from build123d import *

# Parameters (mm, degrees)
SKETCH_1_W          = 120
SKETCH_1_H          = 75
SKETCH_1_W_2        = 114
SKETCH_1_H_2        = 69
EXTRUDE_1_DEPTH     = 45
SKETCH_2_W          = 114
SKETCH_2_H          = 69
SKETCH_2_R          = 30
EXTRUDE_2_DEPTH     = 4
CUT_EXTRUDE_1_DEPTH = 84.852549156
SKETCH_3_W          = 8
SKETCH_3_H          = 8
EXTRUDE_3_DEPTH     = 3
SKETCH_3_3_R        = 0.9
CUT_EXTRUDE_2_DEPTH = 3
SKETCH_4_R          = 5.5
CUT_EXTRUDE_3_DEPTH = 2


with BuildPart() as part:
    # Sketch 1 → Extrude 1 (new body)
    with BuildSketch(Plane.XY):
        Rectangle(SKETCH_1_W, SKETCH_1_H)
        Rectangle(SKETCH_1_W_2, SKETCH_1_H_2, mode=Mode.SUBTRACT)
    extrude(amount=EXTRUDE_1_DEPTH)

    # Sketch 2 → Extrude 2 (add)
    with BuildSketch(Plane.XY.offset(45)):
        Rectangle(SKETCH_2_W, SKETCH_2_H)
        with Locations((-20, 0)):
            Circle(SKETCH_2_R, mode=Mode.SUBTRACT)
    extrude(amount=-EXTRUDE_2_DEPTH)

    # Sketch 2_4 → Cut-Extrude 1 (cut, through all)
    with BuildSketch(Plane.XY.offset(45)):
        with BuildLine():
            ThreePointArc((12.841478126, 8.799847414), (9.44486376, 16.999999947), (4.04163056, 24.04163056))
            ThreePointArc((4.04163056, 24.04163056), (2.415284962, 24.041630558), (2.415284968, 22.41528496))
            ThreePointArc((2.415284968, 22.41528496), (7.453005293, 15.850000012), (10.619848685, 8.204563761))
            ThreePointArc((10.619848685, 8.204563761), (12.02830522, 7.391390911), (12.841478126, 8.799847414))
        make_face()
        with BuildLine():
            ThreePointArc((-28.799847612, -32.841478073), (-20, -34), (-11.200152388, -32.841478073))
            ThreePointArc((-11.200152388, -32.841478073), (-10.386979697, -31.433021385), (-11.795436406, -30.61984873))
            ThreePointArc((-11.795436406, -30.61984873), (-20.000000038, -31.7), (-28.204563667, -30.61984871))
            ThreePointArc((-28.204563667, -30.61984871), (-29.613020313, -31.433021421), (-28.799847612, -32.841478073))
        make_face()
        with BuildLine():
            ThreePointArc((-44.04163056, 24.04163056), (-49.444863704, 17.000000043), (-52.841478068, 8.79984763))
            ThreePointArc((-52.841478068, 8.79984763), (-52.028305318, 7.391390937), (-50.61984868, 8.204563781))
            ThreePointArc((-50.61984868, 8.204563781), (-47.453005293, 15.850000012), (-42.415284981, 22.415284946))
            ThreePointArc((-42.415284981, 22.415284946), (-42.415284955, 24.041630551), (-44.04163056, 24.04163056))
        make_face()
    extrude(amount=-CUT_EXTRUDE_1_DEPTH, mode=Mode.SUBTRACT)

    # Sketch 3 → Extrude 3 (add)
    with BuildSketch(Plane(origin=(0, 0, 0), x_dir=(-1, 0, 0), z_dir=(0, 0, -1))):
        with Locations((-56, 33.5)):
            Rectangle(SKETCH_3_W, SKETCH_3_H)
        with Locations((56, 33.5)):
            Rectangle(SKETCH_3_W, SKETCH_3_H)
        with Locations((-56, -33.5)):
            Rectangle(SKETCH_3_W, SKETCH_3_H)
        with Locations((56, -33.5)):
            Rectangle(SKETCH_3_W, SKETCH_3_H)
    extrude(amount=-EXTRUDE_3_DEPTH)

    # Sketch 3_3 → Cut-Extrude 2 (cut)
    with BuildSketch(Plane(origin=(0, 0, 0), x_dir=(-1, 0, 0), z_dir=(0, 0, -1))):
        with Locations((-56, 33.5)):
            Circle(SKETCH_3_3_R)
        with Locations((-56, -33.5)):
            Circle(SKETCH_3_3_R)
        with Locations((56, -33.5)):
            Circle(SKETCH_3_3_R)
        with Locations((56, 33.5)):
            Circle(SKETCH_3_3_R)
    extrude(amount=-CUT_EXTRUDE_2_DEPTH, mode=Mode.SUBTRACT)

    # Sketch 4 → Cut-Extrude 3 (cut)
    with BuildSketch(Plane.XY.offset(45)):
        with Locations((40, 18)):
            Circle(SKETCH_4_R)
        with Locations((40, 0)):
            Circle(SKETCH_4_R)
        with Locations((40, -18)):
            Circle(SKETCH_4_R)
    extrude(amount=-CUT_EXTRUDE_3_DEPTH, mode=Mode.SUBTRACT)


solid = part.part
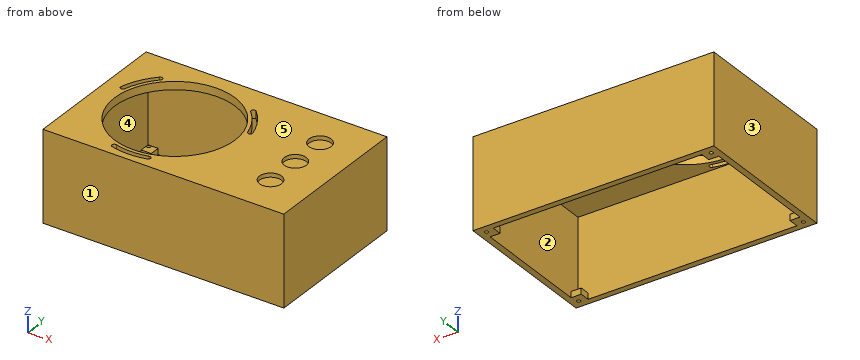
Verification items for the finished model (mm, model axes). Face numbers are marked on the shaded views. A direction names the side the tool comes from. Coordinates: 2 decimals unless noted, no trailing zeros. Order: outer loops, then holes, each group sorted by start corner. A loop starts at its lowest first (then second) coordinate and runs counter-clockwise, first axis right, second up.
Item 1: Access from +Z, -Z, +X, -X, +Y, -Y to the whole of each face (thin tool, end or side, straight path). Record for the marked faces 1 and 2.
Filled in:
face 1: +Z, -Z, +X, -X, -Y
face 2: none
Item 2: Release check for a two-part mould opening along X. For the marked faces 3, 4 and 5 record: +X half, -X half, draft (parallel to the pull), parting line (faces both ways), or undercut.
Filled in:
face 3: -X half
face 4: undercut
face 5: draft
Item 3: Section check D-D, the plane y = 18. Enter the section's corners in (x, z).
Filled in:
outline: (-60, 0) - (-57, 0) - (-57, 41) - (-48.84, 41) - (-48.84, 45) - (-60, 45) - close; (-46.09, 41) - (-44, 41) - (-44, 45) - (-46.09, 45) - close; (4, 41) - (6.09, 41) - (6.09, 45) - (4, 45) - close; (8.84, 41) - (57, 41) - (57, 0) - (60, 0) - (60, 45) - (45.5, 45) - (45.5, 43) - (34.5, 43) - (34.5, 45) - (8.84, 45) - close
Item 4: Section check B-B, the plane z = 33. Enter the section's corners in (x, y).
Filled in:
outline: (-60, -37.5) - (60, -37.5) - (60, 37.5) - (-60, 37.5) - close; hole (-57, -34.5) - (57, -34.5) - (57, 34.5) - (-57, 34.5) - close
Item 5: Material ranges on L1, parallel to Y at x = 40, z = 44; L2, parallel to X at y = 33.5, z = 1.2; L3, parallel to Y at x = -56, z = 2.4, recorded low to high.
Filled in:
L1: y = -37.5 to -23.5, -12.5 to -5.5, 5.5 to 12.5, 23.5 to 37.5
L2: x = -60 to -56.9, -55.1 to -52, 52 to 55.1, 56.9 to 60
L3: y = -37.5 to -34.4, -32.6 to -29.5, 29.5 to 32.6, 34.4 to 37.5
Item 6: Section check C-C, the plane x = -47. Enter the section's corners in (y, z).
Filled in:
outline: (-37.5, 0) - (-34.5, 0) - (-34.5, 41) - (-13.08, 41) - (-13.08, 45) - (-37.5, 45) - close; (13.08, 41) - (16.61, 41) - (16.61, 45) - (13.08, 45) - close; (20.66, 41) - (34.5, 41) - (34.5, 0) - (37.5, 0) - (37.5, 45) - (20.66, 45) - close
Item 7: Section check A-A, the plane y = 0. Enter the section's corners in (x, z).
Filled in:
outline: (-60, 0) - (-57, 0) - (-57, 41) - (-50, 41) - (-50, 45) - (-60, 45) - close; (10, 41) - (57, 41) - (57, 0) - (60, 0) - (60, 45) - (45.5, 45) - (45.5, 43) - (34.5, 43) - (34.5, 45) - (10, 45) - close
Item 8: Depth check by flat-ended pin: pin 1 (9 mm diameter, centred on x = 40, y = 18, fed in from +Z); pin 2 (1.1 mm diameter, centred on x = 56, y = -33.5, fed in from -Z). Enter the tip coordinate at first touch or a pass-through.
Filled in:
pin 1: stops at z = 43
pin 2: stops at z = 41
